```python
from build123d import *

# Parameters (mm, degrees)
SKETCH1_W           = 56
SKETCH1_H           = 48
BOSS_EXTRUDE1_DEPTH = 14
SKETCH3_W           = 50
SKETCH3_H           = 42
CUT_EXTRUDE1_DEPTH  = 12
SKETCH4_R           = 3
SKETCH4_R_2         = 1.5
BOSS_EXTRUDE2_DEPTH = 6
SKETCH5_W           = 22.5
SKETCH5_H           = 12
CUT_EXTRUDE2_DEPTH  = 3
SKETCH6_W           = 12.5
SKETCH6_H           = 10
CUT_EXTRUDE3_DEPTH  = 3
FILLET1_R           = 1
FILLET2_R           = 1


with BuildPart() as part:
    # Sketch1 → Boss-Extrude1 (new body)
    with BuildSketch(Plane(origin=(0, 0, 0), x_dir=(1, 0, 0), z_dir=(0, 1, 0))):
        with Locations((7.929648241, -0.507537688)):
            Rectangle(SKETCH1_W, SKETCH1_H)
    extrude(amount=BOSS_EXTRUDE1_DEPTH)

    # Sketch3 → Cut-Extrude1 (cut)
    with BuildSketch(Plane(origin=(0, 14, 0), x_dir=(1, 0, 0), z_dir=(0, 1, 0))):
        with Locations((7.929648241, -0.507537688)):
            Rectangle(SKETCH3_W, SKETCH3_H)
    extrude(amount=-CUT_EXTRUDE1_DEPTH, mode=Mode.SUBTRACT)

    # Sketch4 → Boss-Extrude2 (add)
    # profile 1 of 4: a face of its own
    with BuildSketch(Plane(origin=(0, 2, 0), x_dir=(1, 0, 0), z_dir=(0, 1, 0))):
        with Locations(Location((-8.070351759, 15.492462312, 0), (0, 0, 270))):
            Circle(SKETCH4_R)
        with Locations(Location((-8.070351759, 15.492462312, 0), (0, 0, 270))):
            Circle(SKETCH4_R_2, mode=Mode.SUBTRACT)
    # profile 2 of 4: a face of its own
    with BuildSketch(Plane(origin=(0, 2, 0), x_dir=(1, 0, 0), z_dir=(0, 1, 0))):
        with Locations(Location((24.929648241, 15.492462312, 0), (0, 0, 270))):
            Circle(SKETCH4_R)
        with Locations(Location((24.929648241, 15.492462312, 0), (0, 0, 270))):
            Circle(SKETCH4_R_2, mode=Mode.SUBTRACT)
    # profile 3 of 4: a face of its own
    with BuildSketch(Plane(origin=(0, 2, 0), x_dir=(1, 0, 0), z_dir=(0, 1, 0))):
        with Locations(Location((24.929648241, -16.757537688, 0), (0, 0, 270))):
            Circle(SKETCH4_R)
        with Locations(Location((24.929648241, -16.757537688, 0), (0, 0, 270))):
            Circle(SKETCH4_R_2, mode=Mode.SUBTRACT)
    # profile 4 of 4: a face of its own
    with BuildSketch(Plane(origin=(0, 2, 0), x_dir=(1, 0, 0), z_dir=(0, 1, 0))):
        with Locations(Location((-8.070351759, -16.757537688, 0), (0, 0, 270))):
            Circle(SKETCH4_R)
        with Locations(Location((-8.070351759, -16.757537688, 0), (0, 0, 270))):
            Circle(SKETCH4_R_2, mode=Mode.SUBTRACT)
    extrude(amount=BOSS_EXTRUDE2_DEPTH)

    # Sketch5 → Cut-Extrude2 (cut)
    with BuildSketch(Plane.ZY.offset(-32.929648241)):
        with Locations((0.507537688, 8)):
            Rectangle(SKETCH5_W, SKETCH5_H)
    extrude(amount=-CUT_EXTRUDE2_DEPTH, mode=Mode.SUBTRACT)

    # Sketch6 → Cut-Extrude3 (cut)
    with BuildSketch(Plane.XY.offset(-20.492462312)):
        with Locations((9.929648241, 9)):
            Rectangle(SKETCH6_W, SKETCH6_H)
    extrude(amount=-CUT_EXTRUDE3_DEPTH, mode=Mode.SUBTRACT)

    # Fillet1
    fillet1_edges = [part.edges().sort_by_distance(p)[0] for p in [
        (34.429648241, 2, -10.742462312),
        (34.429648241, 2, 11.757537688),
        (3.679648241, 4, -21.992462312),
        (16.179648241, 4, -21.992462312),
    ]]
    fillet(fillet1_edges, radius=FILLET1_R)

    # Fillet2
    fillet2_edges = [part.edges().sort_by_distance(p)[0] for p in [
        (-8.070351759, 2, -18.492462312),
        (24.929648241, 2, -18.492462312),
        (24.929648241, 2, 13.757537688),
        (-8.070351759, 2, 13.757537688),
    ]]
    fillet(fillet2_edges, radius=FILLET2_R)


solid = part.part
```
For this review, take the finished solid that the model builds, in its own axes (mm). A direction names the side the tool comes from. Coordinates: 2 decimals unless noted, no trailing zeros. Write each loop counter-clockwise with the first axis right and the second up, starting at its lowest first coordinate (ties: lowest second). Pieces come first, ordered by that corner, then holes.
(1) For pin 1 Ø5 at (x, z) = (-11.5, -13.5) entering from -Y; pin 2 Ø6 at (y, z) = (10.5, 5.5) entering from +X; pin 3 Ø5 at (x, z) = (-12.5, -6.5) entering from +Y; pin 4 Ø5 at (x, z) = (24.93, 16.76) entering from +Y, all flat-tipped, find the tip position at first contact; note any pin that passes through.
(2) Add section B-B on x = 13.5. Give the boundary of the cut face in (y, z), then the cut area to 3 significant figures.
(3) Wall thickness on probe 1 along Z at (x, y) = (-2, 6.75); probe 2 along Z at (x, y) = (33, 12.5); probe 3 along X at (y, z) = (6.75, 19.5): over which ranges is each line inside the solid? List them lowest first.
(4) Add section C-C on z = -1.5. Give the boundary of the cut face in (x, y), then the cut area to 3 significant figures.
(5) Add section D-D on x = -14. Give the boundary of the cut face in (y, z), then the cut area to 3 significant figures.
(6) Add section A-A on y = 10.25. Give the boundary of the cut face in (x, z), then the cut area to 3 significant figures.
(7) The part is to be moulded in two halves that separate along Z. For faces 4 (the face through (34, 8, 11.758)), 5 (the face through (26.194, 4.958, -14.686)), 6 (the face through (3.68, 9, -22)), 7 (the face through (8, 7, 24.508)), say which applies: +Z half, -Z half, draft (parallel to the pull), parting line (faces both ways), or undercut.
(8) Tool access review of faces 1 (the face through (34, 8, -10.742)), 2 (the face through (25, 2, 17)), 3 (the face through (10, 4, -22)): name each direction out of +Z, -Z, +X, -X, +Y, -Y from which nothing blocks a thin tool from reaching the whole face with its end or side.
Answer sheet:
1. pin 1: stops at y = 0
1. pin 2: stops at x = -17.07
1. pin 3: stops at y = 2
1. pin 4: stops at y = 8
2. outline: (0, -23.49) - (4, -23.49) - (4, -20.49) - (2, -20.49) - (2, 21.51) - (14, 21.51) - (14, 24.51) - (0, 24.51) - close
2. area: 138 mm2
3. probe 1: z = -23.49 to -20.49, 21.51 to 24.51
3. probe 2: z = -23.49 to -10.74, 11.76 to 24.51
3. probe 3: x = -20.07 to -17.07, -9.29 to -6.85, 23.71 to 26.15, 32.93 to 35.93
4. outline: (-20.07, 0) - (35.93, 0) - (35.93, 2) - (-17.07, 2) - (-17.07, 14) - (-20.07, 14) - close
4. area: 148 mm2
5. outline: (0, -23.49) - (14, -23.49) - (14, -20.49) - (2, -20.49) - (2, 21.51) - (14, 21.51) - (14, 24.51) - (0, 24.51) - close
5. area: 168 mm2
6. outline: (-20.07, -23.49) - (3.68, -23.49) - (3.68, -20.49) - (-17.07, -20.49) - (-17.07, 21.51) - (32.93, 21.51) - (32.93, 11.76) - (35.93, 11.76) - (35.93, 24.51) - (-20.07, 24.51) - close; (16.18, -23.49) - (35.93, -23.49) - (35.93, -10.74) - (32.93, -10.74) - (32.93, -20.49) - (16.18, -20.49) - close
6. area: 483 mm2
7. face 4: undercut
7. face 5: undercut
7. face 6: draft
7. face 7: +Z half
8. face 1: +X, +Y
8. face 2: +Y
8. face 3: -Z, +Y
